The listing builds one solid part. Answer for the finished solid, in the listing's coordinates (mm). A direction names the side the tool comes from. Give positions to 0.01 mm unless a question says otherwise; leave off trailing zeros. Order: outer loops, then holes, each group sorted by start corner. A loop starts at its lowest first (then second) coordinate and runs counter-clockwise, first axis right, second up. Notation, with made-up numbers: (10.5, 29) - (44.5, 29) arc R29 cw to (44.5, 56) - close; hole circle Ø11 at (3.25, 79). An arc over 180 degrees is marked (long way). Answer as CSV lines item,"result". Start each with the question number.
1. Which of the six approach directions +Z, -Z, +X, -X, +Y, -Y give full straight-line access (tool end or side, diameter ignored) to faces 1 (the cylindrical face through (63, 15, 0)), 2 (the cylindrical face through (65, 14, 0)), 3 (the flat face through (24, 15, -4))?
2. Section C-C on y = 14.5 is taken. Give the vertices of the cut face in (x, z), and give its area (3 significant figures).
3. Section D-D on x = 20 is taken. Give the vertices of the cut face in (y, z).
4. Flat-ended cylindrical pins translate along their axes: pin 1 (0.6 mm diameter, centred on y = 20.5, z = -4, fed in from -X); pin 2 (2 mm diameter, centred on x = 24, z = 0, fed in from +Y); pin 3 (0.6 mm diameter, centred on y = 13, z = -4.5, fed in from +X). Find the tip coordinate at first contact, or state that the pin passes through.
5. Section B-B on x = 53 is taken. Give the vertices of the cut face in (y, z).
6. Consider line 1 along Z through (x, y) = (-11.5, 26.5); line 2 along X through (y, z) = (24.5, -0.25); line 3 along Y through (x, z) = (32.5, 2.25). Determine where each line is inside the solid, lowest interval first. Write a range as [from, to].
7. Section A-A on z = -4 is taken. Give the vertices of the cut face in (x, y), and give its area (3 significant figures).
8. Determine the mould class of faces 4 (the cylindrical face through (-25, 14, 0)), 5 (the flat face through (-2, 15, -3)), 6 (the flat face through (11, 14, -5)) for opening direction X: +X half, -X half, draft (parallel to the pull), parting line (faces both ways), or undercut.
from build123d import *

# Parameters (mm, degrees)
EXTRUDE_1_DEPTH     = 30
EXTRUDE_2_DEPTH     = 2
SKETCH_3_W          = 8
SKETCH_3_H          = 2.352392564
CUT_EXTRUDE_1_DEPTH = 30


with BuildPart() as part:
    # 草圖1 → 填料-伸長1 (new body)
    with BuildSketch(Plane(origin=(0, 0, 0), x_dir=(1, 0, 0), z_dir=(0, 1, 0))):
        with BuildLine():
            Line((-20, 5), (60, 5))
            ThreePointArc((60, 5), (65, 0), (60, -5))
            Line((60, -5), (-20, -5))
            ThreePointArc((-20, -5), (-25, 0), (-20, 5))
        make_face()
        with BuildLine():
            Line((-20, 3), (60, 3))
            ThreePointArc((60, 3), (63, 0), (60, -3))
            Line((60, -3), (-20, -3))
            ThreePointArc((-20, -3), (-23, 0), (-20, 3))
        make_face(mode=Mode.SUBTRACT)
    extrude(amount=EXTRUDE_1_DEPTH)

    # 草圖2 → 填料-伸長2 (add)
    with BuildSketch(Plane.XZ):
        with BuildLine():
            Line((-20, -5), (60, -5))
            ThreePointArc((60, -5), (65, 0), (60, 5))
            Line((60, 5), (-20, 5))
            ThreePointArc((-20, 5), (-25, 0), (-20, -5))
        make_face()
    extrude(amount=EXTRUDE_2_DEPTH)

    # 草圖3 → 除料-伸長1 (cut)
    with BuildSketch(Plane(origin=(0, 30, 0), x_dir=(1, 0, 0), z_dir=(0, 1, 0))):
        with Locations((20, 3.823803718)):
            Rectangle(SKETCH_3_W, SKETCH_3_H)
    extrude(amount=-CUT_EXTRUDE_1_DEPTH, mode=Mode.SUBTRACT)


solid = part.part
Checks:
1,face 1,"+Y"
1,face 2,"+X, +Y, -Y"
1,face 3,"-Z, +Y"
2,outline,"(-20, -5) - (16, -5) - (16, -3) - (-20, -3) arc R3 cw to (-20, 3) - (60, 3) arc R3 cw to (60, -3) - (24, -3) - (24, -5) - (60, -5) arc R5 ccw to (60, 5) - (-20, 5) arc R5 ccw to start"
2,area,"354 mm²"
3,outline,"(-2, -5) - (0, -5) - (0, 3) - (30, 3) - (30, 5) - (-2, 5) - close"
4,pin 1,"stops at x = -23.36"
4,pin 2,"stops at y = 0"
4,pin 3,"stops at x = 62.71"
5,outline,"(-2, -5) - (30, -5) - (30, -3) - (0, -3) - (0, 3) - (30, 3) - (30, 5) - (-2, 5) - close"
6,line 1,"z = [-5, -3], [3, 5]"
6,line 2,"x = [-24.99, -22.99], [62.99, 64.99]"
6,line 3,"y = [-2, 0]"
7,outline,"(-23, -2) - (63, -2) - (63, 30) - (24, 30) - (24, 0) - (16, 0) - (16, 30) - (-23, 30) - close"
7,area,"2,510 mm²"
8,face 4,"-X half"
8,face 5,"undercut"
8,face 6,"draft"
